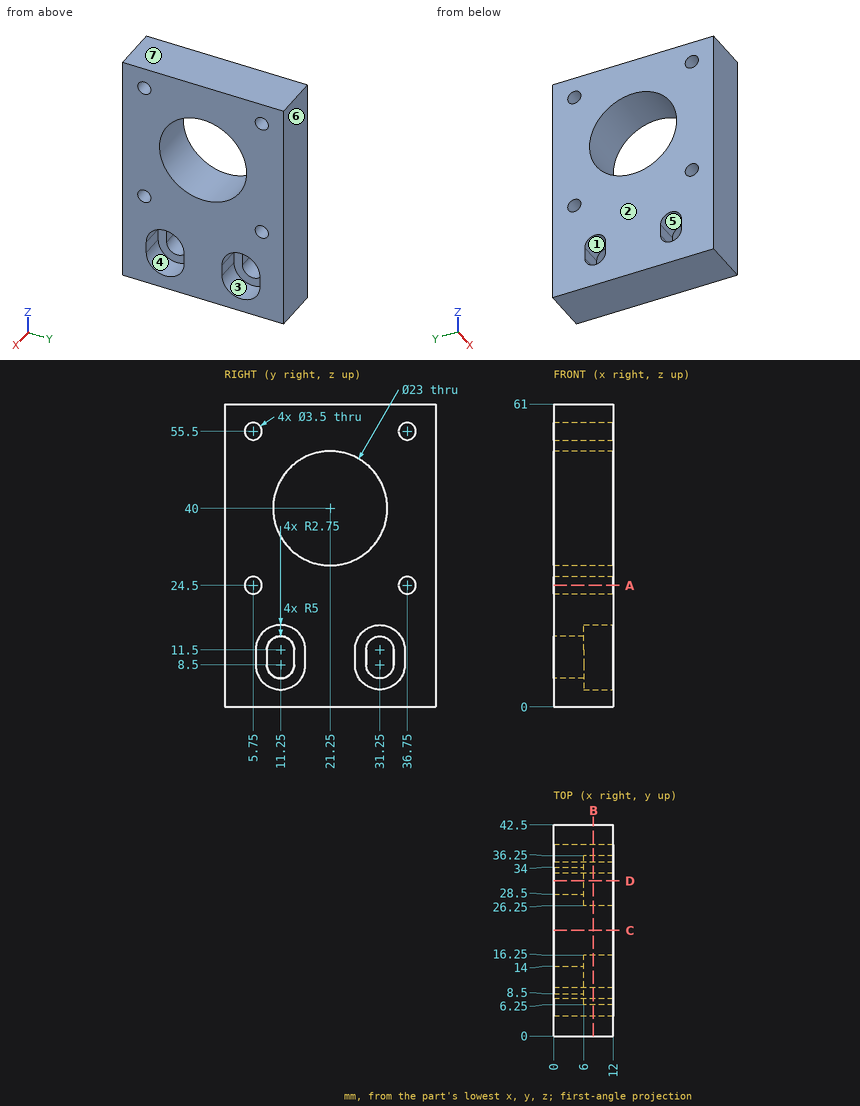
Input: dimensioned drawing with shaded views. Units: mm. Origin: part minimum x, y, z. A direction names the side the tool comes from. Round coordinates to 2 decimals unless told otherwise and drop trailing zeros. Order: outer loops, then holes, each group sorted by start corner. A loop starts at its lowest first (then second) coordinate and runs counter-clockwise, first axis right, second up.
1. Cut plane C-C, the plane y = 21.25. Output: boundary loops of the cut face in (x, z).
The answers:
outline: (0, 0) - (12, 0) - (12, 28.5) - (0, 28.5) - close; (0, 51.5) - (12, 51.5) - (12, 61) - (0, 61) - close
2. Cut plane B-B, the plane x = 8. Output: boundary loops of the cut face in (y, z), then the cut area to 3 significant figures.
The answers:
outline: (0, 0) - (42.5, 0) - (42.5, 61) - (0, 61) - close; hole circle Ø3.5 at (5.75, 24.5); hole circle Ø3.5 at (5.75, 55.5); hole (6.25, 8.5) arc R5 ccw to (16.25, 8.5) - (16.25, 11.5) arc R5 ccw to (6.25, 11.5) - close; hole circle Ø23 at (21.25, 40); hole (26.25, 8.5) arc R5 ccw to (36.25, 8.5) - (36.25, 11.5) arc R5 ccw to (26.25, 11.5) - close; hole circle Ø3.5 at (36.75, 24.5); hole circle Ø3.5 at (36.75, 55.5)
area: 1,920 mm2
3. Pin query (flat end, axial travel): P1, Ø20.5, axis at y = 21.25, z = 40, coming from the +X side. Return the tip coordinate at first contact, or that it passes through.
The answers:
P1: passes through
4. Material intervals for line 1 (Y direction, x = 3.5, z = 24.5); line 2 (Y direction, x = 3, z = 11); line 3 (Z direction, x = 9.5, y = 14.5), sorted ascending.
The answers:
line 1: y = 0 to 4, 7.5 to 35, 38.5 to 42.5
line 2: y = 0 to 8.5, 14 to 28.5, 34 to 42.5
line 3: z = 0 to 4.7, 15.3 to 30.69, 49.31 to 61
5. Cut plane A-A, the plane z = 24.5. Output: boundary loops of the cut face in (x, y).
The answers:
outline: (0, 0) - (12, 0) - (12, 4) - (0, 4) - close; (0, 7.5) - (12, 7.5) - (12, 35) - (0, 35) - close; (0, 38.5) - (12, 38.5) - (12, 42.5) - (0, 42.5) - close
6. Mould query, pull axis Y, two halves, no side actions, for the marked faces 4, 5, 6 and 7. Classes: released by +Y, released by -Y, zero draft, split by the parting line, or undercut.
The answers:
face 4: undercut
face 5: undercut
face 6: released by +Y
face 7: zero draft
7. Set-up query: the marked faces 1, 2 and 3. Return all of +Z, -Z, +X, -X, +Y, -Y with unobstructed straight access to the full face (end or side cutting, diameter ignored); none if empty.
The answers:
face 1: +X, -X
face 2: +Z, -Z, -X, +Y, -Y
face 3: +X
8. Cut plane D-D, the plane y = 31.25. Output: boundary loops of the cut face in (x, z).
The answers:
outline: (0, 0) - (12, 0) - (12, 3.5) - (6, 3.5) - (6, 5.75) - (0, 5.75) - close; (0, 14.25) - (6, 14.25) - (6, 16.5) - (12, 16.5) - (12, 34.32) - (0, 34.32) - close; (0, 45.68) - (12, 45.68) - (12, 61) - (0, 61) - close
